Work out the finished part from the listing and answer in its coordinate system (mm). Face numbers are marked on the shaded views. A direction names the side the tool comes from. Round coordinates to 2 decimals unless told otherwise and drop trailing zeros. Write each loop counter-clockwise with the first axis right and the second up, starting at its lowest first coordinate (ties: lowest second). Pieces come first, ordered by that corner, then holes. Notation, with made-up numbers: (43, -30.5) - (89, -30.5) arc R18 ccw to (89, -21.5) - close; hole circle Ø7 at (38, 34). An arc over 180 degrees is marked (long way). Answer as a JSON object with one key per item and string values.
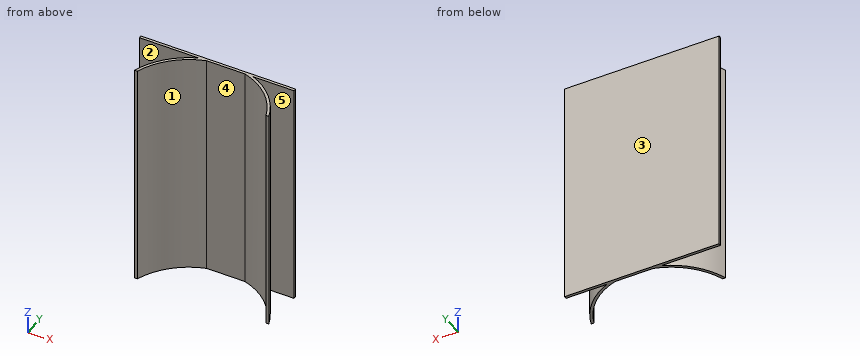
```python
from build123d import *

# Parameters (mm, degrees)
ESQUISSE1_W        = 170
ESQUISSE1_H        = 3
BOSS_EXTRU_1_DEPTH = 250
BOSS_EXTRU_2_DEPTH = 250


with BuildPart() as part:
    # Esquisse1 → Boss.-Extru.1 (new body)
    with BuildSketch(Plane.XY):
        with Locations((85, 1.5)):
            Rectangle(ESQUISSE1_W, ESQUISSE1_H)
    extrude(amount=BOSS_EXTRU_1_DEPTH)

    # Esquisse3 → Boss.-Extru.2 (add)
    with BuildSketch(Plane.XY.offset(250)):
        with BuildLine():
            Line((21.114954152, -47), (24.289321881, -47))
            ThreePointArc((24.289321881, -47), (43.473675463, -17.501946092), (74, 0))
            Line((74, 0), (65, 0))
            ThreePointArc((65, 0), (37.988810855, -18.767262777), (21.114954152, -47))
        make_face()
        with BuildLine():
            Line((165.710678119, -47), (168.885045848, -47))
            ThreePointArc((168.885045848, -47), (152.011189145, -18.767262777), (125, 0))
            Line((125, 0), (116, 0))
            ThreePointArc((116, 0), (146.526324537, -17.501946092), (165.710678119, -47))
        make_face()
    extrude(amount=-BOSS_EXTRU_2_DEPTH)


solid = part.part
```
Item 1: Determine the mould class of the marked faces 4 and 5 for opening direction X: pulls with the +X half, pulls with the -X half, needs draft (parallel to the pull), parting line crosses it, or undercut.
Results found:
{"face 4": "undercut", "face 5": "needs draft"}
Item 2: A cutting plane is placed at C-C (z = 177). Write down the section's boundary in (x, y), and give its area (3 significant figures).
Results found:
{"outline": "(0, 0) - (65, 0) arc R78 ccw to (21.11, -47) - (24.29, -47) arc R75 cw to (74, 0) - (116, 0) arc R75 cw to (165.71, -47) - (168.89, -47) arc R78 ccw to (125, 0) - (170, 0) - (170, 3) - (0, 3) - close", "area": "921 mm²"}
Item 3: For the marked faces 1, 2 and 3, determine the directions among +Z, -Z, +X, -X, +Y, -Y from which every point of the face is accessible in a straight line to the end or side of a thin tool.
Results found:
{"face 1": "+Z, -Z, -Y", "face 2": "+Z, -Z, -X", "face 3": "+Z, -Z, +X, -X, +Y"}
Item 4: Each of these flat-tipped pins is pushed along its axis until it touches: P1, Ø12, axis at y = -9, z = 163.5, coming from the +X side; P2, Ø10, axis at y = -8, z = 136, coming from the +X side; P3, Ø6, axis at y = -30.5, z = 54, coming from the +X side. Where does it stop, or does it pass through?
Results found:
{"P1": "x = 148.24", "P2": "x = 146.02", "P3": "x = 162.84"}
Item 5: A cutting plane is placed at D-D (x = 111.5). Write down the section's boundary in (y, z), and give its area (3 significant figures).
Results found:
{"outline": "(0, 0) - (3, 0) - (3, 250) - (0, 250) - close", "area": "750 mm²"}
Item 6: A cutting plane is placed at A-A (x = 159). Write down the section's boundary in (y, z).
Results found:
{"outline": "(-32.9, 0) - (-27.41, 0) - (-27.41, 250) - (-32.9, 250) - close; (0, 0) - (3, 0) - (3, 250) - (0, 250) - close"}
Item 7: Consider line 1 along Y through (x, z) = (19.5, 127.5); line 2 along X through (y, z) = (-35, 64); line 3 along Y through (x, z) = (40.5, 20.5). Determine where each line is inside the solid, lowest interval first.
Results found:
{"line 1": "0 to 3", "line 2": "26.33 to 29.76, 160.24 to 163.67", "line 3": "-20.48 to -16.2, 0 to 3"}
Item 8: A cutting plane is placed at B-B (y = -21). Write down the section's boundary in (x, z).
Results found:
{"outline": "(35.98, 0) - (40.01, 0) - (40.01, 250) - (35.98, 250) - close; (149.99, 0) - (154.02, 0) - (154.02, 250) - (149.99, 250) - close"}
